Design review of the part built by this model. Coordinates are the model's own, in mm. Give positions to 0.01 mm unless a question says otherwise; leave off trailing zeros. Write each loop counter-clockwise with the first axis right and the second up, starting at its lowest first coordinate (ties: lowest second). Pieces come first, ordered by that corner, then holes.
```python
from build123d import *

# Parameters (mm, degrees)
F0_W     = 20.32
F0_H     = 12.7
F0_W_2   = 0.6
F0_H_2   = 0.6
F0_R     = 1.0922
F1_DEPTH = 1


with BuildPart() as f1:
    # F0 (on Top) → F1 (new body)
    with BuildSketch(Plane.XY):
        with Locations((10.16, 6.35)):
            Rectangle(F0_W, F0_H)
        with Locations((1.25, 1.35)):
            Rectangle(F0_W_2, F0_H_2, mode=Mode.SUBTRACT)
        with Locations((1.25, 3.85)):
            Rectangle(F0_W_2, F0_H_2, mode=Mode.SUBTRACT)
        with Locations((1.25, 6.35)):
            Rectangle(F0_W_2, F0_H_2, mode=Mode.SUBTRACT)
        with Locations((3.75, 6.35)):
            Rectangle(F0_W_2, F0_H_2, mode=Mode.SUBTRACT)
        with Locations((1.25, 8.85)):
            Rectangle(F0_W_2, F0_H_2, mode=Mode.SUBTRACT)
        with Locations((1.25, 11.35)):
            Rectangle(F0_W_2, F0_H_2, mode=Mode.SUBTRACT)
        with Locations((17.78, 10.16)):
            Circle(F0_R, mode=Mode.SUBTRACT)
    extrude(amount=F1_DEPTH)


solid = f1.part
```
(1) To check wall thickness, follow L1, parallel to Y at x = 17.78, z = 0.5; L2, parallel to X at y = 6.25, z = 0.5; L3, parallel to Y at x = 4, z = 0.2. State the ranges of each line that lie inside material, in increasing order.
Resolved:
L1: y = 0 to 9.07, 11.25 to 12.7
L2: x = 0 to 0.95, 1.55 to 3.45, 4.05 to 20.32
L3: y = 0 to 6.05, 6.65 to 12.7
(2) Mouldability with a two-part tool opening along X and no side actions: class faces 1 (the face through (10, 6, 1)), 2 (the face through (20.32, 6.3, 0.5)), 3 (the face through (16.975, 10.898, 0.493)) as pulls with the +X half, pulls with the -X half, needs draft (parallel to the pull), parting line crosses it, or undercut.
Resolved:
face 1: needs draft
face 2: pulls with the +X half
face 3: undercut
(3) Consider section C-C, the plane z = 0.2. Give the number of separate pieces and of enclosed holes in the cut face, then the cut area to 3 significant figures.
Resolved:
separate pieces: 1
enclosed holes: 7
area: 252 mm2
(4) Consider section A-A, the plane y = 10.16. Give the boundary of the cut face in (x, z).
Resolved:
outline: (0, 0) - (16.69, 0) - (16.69, 1) - (0, 1) - close; (18.87, 0) - (20.32, 0) - (20.32, 1) - (18.87, 1) - close
(5) Consider section B-B, the plane x = 17.78. Give the boundary of the cut face in (y, z).
Resolved:
outline: (0, 0) - (9.07, 0) - (9.07, 1) - (0, 1) - close; (11.25, 0) - (12.7, 0) - (12.7, 1) - (11.25, 1) - close
